Check sheet for the modelled part. Datum: model origin and axes. Units: mm. A direction names the side the tool comes from. Give positions to 0.01 mm unless a question says otherwise; leave off trailing zeros. Loops run counter-clockwise (first coordinate to the right, second up) from the corner with the lowest first, then second, coordinate; pieces in that order, holes last. Notation, with made-up numbers: M 65,3.25 L 85,3.25 A6 cw 85,8.25 Z; hole C -24,59.5 d10. An arc over 180 degrees is marked long. Write each question's results on one line, items separated by ' | '. Start each with the question number.
1. Go/stop test with flat-tipped pins: pin 1 (1 mm diameter, centred on x = 17.5, z = 1.5, fed in from +Y); pin 2 (1.8 mm diameter, centred on y = 8.5, z = 6, fed in from +X); pin 3 (1.8 mm diameter, centred on y = 9.5, z = 3.5, fed in from -X). Record where each tip stops, or that it passes through.
2. Sectioned sample at C-C on x = 8. Record the cut outline in (y, z), and give its area (3 significant figures).
3. Sectioned sample at A-A on y = -3. Record the cut outline in (x, z), and give its area (3 significant figures).
4. Material ranges on line 1 along X through (y, z) = (-1.5, 6.25); line 2 along Z through (x, y) = (12, 7.5); line 3 along Y through (x, z) = (0, 5.5), recorded low to high.
5. Draft check along Z on faces 6 (the cylindrical face through (14.6, 4.5, 5.1)), 7 (the cylindrical face through (12.86, 4.395, 3.385)), 8 (the flat face through (3, -2, 5)), 9 (the flat face through (-2, 0, 10)). Enter one of: pulls with the +Z half, pulls with the -Z half, needs draft (parallel to the pull), parting line crosses it, or undercut.
6. Sectioned sample at D-D on y = 8.5. Record the cut outline in (x, z), and give its area (3 significant figures).
7. Sectioned sample at B-B on z = 5. Record the cut outline in (x, y), and give its area (3 significant figures).
8. Tool access check on faces 1 (the flat face through (0, 0, 0)), 2 (the flat face through (0, 7.5, 5)), 3 (the flat face through (6, 8, 5)), 4 (the flat face through (-1.5, 0, 7)), 5 (the flat face through (23, 5, 7)). Record the directions out of +Z, -Z, +X, -X, +Y, -Y that give a thin tool (end or side, any length) a straight path to the whole face; none if there is none.
```python
from build123d import *

# Parameters (mm, degrees)
SKETCH1_W           = 6
SKETCH1_H           = 15
BOSS_EXTRUDE1_DEPTH = 10
SKETCH2_W           = 3
SKETCH2_H           = 10
CUT_EXTRUDE1_DEPTH  = 7
SKETCH3_R           = 3.5
BOSS_EXTRUDE2_DEPTH = 20
SKETCH5_R           = 3
CUT_EXTRUDE2_DEPTH  = 17
SKETCH6_W           = 2.5
SKETCH6_H           = 1
CUT_EXTRUDE3_DEPTH  = 17


with BuildPart() as part:
    # Sketch1 → Boss-Extrude1 (new body)
    with BuildSketch(Plane.XY):
        Rectangle(SKETCH1_W, SKETCH1_H)
    extrude(amount=BOSS_EXTRUDE1_DEPTH)

    # Sketch2 → Cut-Extrude1 (cut)
    with BuildSketch(Plane.XY.offset(10)):
        Rectangle(SKETCH2_W, SKETCH2_H)
    extrude(amount=-CUT_EXTRUDE1_DEPTH, mode=Mode.SUBTRACT)

    # Sketch3 → Boss-Extrude2 (add)
    with BuildSketch(Plane(origin=(3, 0, 0), x_dir=(0, 0, -1), z_dir=(1, 0, 0))):
        with Locations((-5, 7.5)):
            Circle(SKETCH3_R)
    extrude(amount=BOSS_EXTRUDE2_DEPTH)

    # Sketch5 → Cut-Extrude2 (cut)
    with BuildSketch(Plane(origin=(23, 0, 0), x_dir=(0, 0, -1), z_dir=(1, 0, 0))):
        with Locations(Location((-5, 7.5, 0), (0, 0, 90))):
            Circle(SKETCH5_R)
    extrude(amount=-CUT_EXTRUDE2_DEPTH, mode=Mode.SUBTRACT)

    # Sketch6 → Cut-Extrude3 (cut)
    with BuildSketch(Plane(origin=(23, 0, 0), x_dir=(0, 0, -1), z_dir=(1, 0, 0))):
        with Locations((-5, 10.5)):
            Rectangle(SKETCH6_W, SKETCH6_H)
    extrude(amount=-CUT_EXTRUDE3_DEPTH, mode=Mode.SUBTRACT)


solid = part.part
```
Output values:
1) pin 1: y = 9.3 | pin 2: x = 6 | pin 3: x = 3
2) outline: M 10.23,3.75 A3 cw long 10.23,6.25 L 10.77,6.25 A3.5 ccw long 10.77,3.75 Z | area: 8.93 mm2
3) outline: M -3,0 L 3,0 L 3,10 L 1.5,10 L 1.5,3 L -1.5,3 L -1.5,10 L -3,10 Z | area: 39.0 mm2
4) line 1: -3 to -1.5, 1.5 to 3 | line 2: 1.5 to 2, 8 to 8.5 | line 3: -7.5 to -5, 5 to 7.5
5) face 6: undercut | face 7: parting line crosses it | face 8: needs draft | face 9: pulls with the +Z half
6) outline: M 3,1.65 L 23,1.65 L 23,2.17 L 6,2.17 L 6,7.83 L 23,7.83 L 23,8.35 L 3,8.35 Z | area: 38.0 mm2
7) outline: M -3,-7.5 L 3,-7.5 L 3,4 L 23,4 L 23,4.5 L 6,4.5 L 6,11 L 3,11 L 3,7.5 L -3,7.5 Z; hole M -1.5,-5 L 1.5,-5 L 1.5,5 L -1.5,5 Z | area: 89.5 mm2
8) face 1: -Z, +X, -X, +Y, -Y | face 2: +Z, -Z, -X, +Y | face 3: +X | face 4: +Z | face 5: +Z, -Z, +X, +Y, -Y
